Verification items for the finished model (mm, model axes). A direction names the side the tool comes from. Round coordinates to 2 decimals unless told otherwise and drop trailing zeros. Order: outer loops, then holes, each group sorted by start corner. A loop starts at its lowest first (then second) coordinate and runs counter-clockwise, first axis right, second up.
Autodesk Inventor part; units mm, degrees
ref_plane "YZ Plane" through (0, 0, 0) normal (1, 0, 0) x (0, 1, 0)
ref_plane "XZ Plane" through (0, 0, 0) normal (0, 1, 0) x (-1, 0, 0)
ref_plane "XY Plane" through (0, 0, 0) normal (0, 0, 1) x (1, 0, 0)
sketch "スケッチ1" plane through (0, 0, 0) normal (0, 0, 1) x (1, 0, 0)
  circle A0 centre (0, 0) radius 3
  dimension "d0" = 6
extrude "押し出し1" add sketch "スケッチ1" along normal blind 45
sketch "スケッチ2" plane through (0, 0, 45) normal (0, 0, 1) x (1, 0, 0)
  circle A0 centre (0, 0) radius 3
  circle A1 centre (0, 0) radius 1.25
  dimension "d3" = 2.5
extrude "押し出し2" cut sketch "スケッチ2" against normal blind 6 contours A1
sketch "スケッチ3" plane through (0, 0, 0) normal (0, 0, -1) x (-1, 0, 0)
  circle A0 centre (0, 0) radius 3
  circle A1 centre (0, 0) radius 1.25
  dimension "d6" = 2.5
extrude "押し出し3" cut sketch "スケッチ3" against normal blind 6 contours A1
sketch "スケッチ4" plane through (0, 0, 45) normal (0, 0, 1) x (1, 0, 0)
  circle A0 centre (0, 0) radius 1.25
  circle A1 centre (0, 0) radius 3
extrude "押し出し4" cut sketch "スケッチ4" against normal blind 5
sketch "スケッチ5" plane through (0, 0, 40) normal (0, 0, 1) x (1, 0, 0)
  circle A0 centre (0, 0) radius 1.25
extrude "押し出し5" cut sketch "スケッチ5" against normal blind 6
sketch "スケッチ6" plane through (0, 0, 40) normal (0, 0, 1) x (1, 0, 0)
  circle A0 centre (0, 0) radius 1.25
extrude "押し出し6" add sketch "スケッチ6" along normal mid plane 12
properties part number "φ6スペーサ　L40　おねめじ" material "Aluminum-6061"
1) Tool access check on faces 4 (the cylindrical face through (0.27, -1.22, 2.96)), 5 (the flat face through (1, -1, 0)). Record the directions out of +Z, -Z, +X, -X, +Y, -Y that give a thin tool (end or side, any length) a straight path to the whole face; none if there is none.
2) Sectioned sample at C-C on z = 38.5. Record the cut outline in (x, y).
3) Sectioned sample at A-A on y = 0. Record the cut outline in (x, z), then the cut area to 3 significant figures.
4) Sectioned sample at D-D on y = -2.55. Record the cut outline in (x, z), then the cut area to 3 significant figures.
5) Scan lines: probe 1 along Y at (x, z) = (0, 3.85); probe 2 along X at (y, z) = (0.2, 30); probe 3 along Z at (x, y) = (1.35, -0.1). Record each from-to range of solid material in increasing order.
6) Go/stop test with flat-tipped pins: pin 1 Ø1 at (y, z) = (2, 13.5) entering from +X; pin 2 Ø1 at (y, z) = (2.5, 21.5) entering from +X; pin 3 Ø1.5 at (x, y) = (0, 0) entering from -Z. Record where each tip stops, or that it passes through.
7) Draft check along X on faces 1 (the cylindrical face through (-0.27, 1.22, 42.96)), 2 (the flat face through (1, -1, 40)), 3 (the flat face through (0, 0, 6)). Enter one of: released by +X, released by -X, zero draft, split by the parting line, or undercut.
Returned:
1. face 4: -Z
1. face 5: -Z, +X, -X, +Y, -Y
2. outline: circle Ø6 at (0, 0)
3. outline: (-3, 0) - (-1.25, 0) - (-1.25, 6) - (1.25, 6) - (1.25, 0) - (3, 0) - (3, 40) - (1.25, 40) - (1.25, 46) - (-1.25, 46) - (-1.25, 40) - (-3, 40) - close
3. area: 240 mm2
4. outline: (-1.58, 0) - (1.58, 0) - (1.58, 40) - (-1.58, 40) - close
4. area: 126 mm2
5. probe 1: y = -3 to -1.25, 1.25 to 3
5. probe 2: x = -2.99 to 2.99
5. probe 3: z = 0 to 40
6. pin 1: stops at x = 2.6
6. pin 2: stops at x = 2.24
6. pin 3: stops at z = 6
7. face 1: split by the parting line
7. face 2: zero draft
7. face 3: undercut
